from build123d import *

# Parameters (mm, degrees)
F0_R     = 1.4605
F1_DEPTH = 6.35


# Not quite as in the source:
# - a feature names something its author has since deleted; it is built from what else it names


with BuildPart() as f1:
    # F0 (on Top) → F1 (new body)
    with BuildSketch(Plane.XY):
        Polygon((76.2, 19.05), (76.2, 35.8597988734), (-76.2, 35.8597988734), (-76.2, 21.2902011266), (-73.2282, 21.2902011266), (-73.2282, 1.4605), (-65.6082, 1.4605), (-65.6082, 3.175), (-63.1952, 3.175), (-63.1952, 1.4605), (-55.5752, 1.4605), (-55.5752, -1.4605), (-63.1952, -1.4605), (-63.1952, -3.175), (-65.6082, -3.175), (-65.6082, -1.4605), (-73.2282, -1.4605), (-73.2282, -16.8097988734), (-76.2, -16.8097988734), (-76.2, -35.8597988734), (-57.15, -35.8597988734), (-57.15, -38.8315988734), (-19.05, -38.8315988734), (-19.05, -35.8597988734), (-1.4605, -35.8597988734), (-1.4605, -28.2397988734), (-3.175, -28.2397988734), (-3.175, -25.8267988734), (-1.4605, -25.8267988734), (-1.4605, -18.2067988734), (1.4605, -18.2067988734), (1.4605, -25.8267988734), (3.175, -25.8267988734), (3.175, -28.2397988734), (1.4605, -28.2397988734), (1.4605, -35.8597988734), (19.05, -35.8597988734), (19.05, -38.8315988734), (57.15, -38.8315988734), (57.15, -36.9798994367), (57.15, -35.8597988734), (76.2, -35.8597988734), (76.2, -19.05), (73.2282, -19.05), (73.2282, -1.4605), (65.6082, -1.4605), (65.6082, -3.175), (63.1952, -3.175), (63.1952, -1.4605), (55.5752, -1.4605), (55.5752, 1.4605), (63.1952, 1.4605), (63.1952, 3.175), (65.6082, 3.175), (65.6082, 1.4605), (73.2282, 1.4605), (73.2282, 19.05), align=None)
        with Locations((-38.1, -37.3456988734)):
            Circle(F0_R, mode=Mode.SUBTRACT)
        with BuildLine():
            ThreePointArc((39.5605, -37.3456988734), (39.5181253393, -37.6949563314), (39.3934602575, -38.0239472145))
            ThreePointArc((39.3934602575, -38.0239472145), (36.6818746607, -36.9964414154), (39.5605, -37.3456988734))
        make_face(mode=Mode.SUBTRACT)
        with BuildLine():
            add(Edge.make_bspline(
                [(-21.3872035351, 27.8586064071), (-20.0222567073, 26.4936595793), (-20.0222567073, 24.0434586691)],
                knots=[0, 0, 0, 1, 1, 1], degree=2))
            add(Edge.make_bspline(
                [(-20.0222567073, 24.0434586691), (-20.0222567073, 21.4291405282), (-21.441524027, 20.0457016181)],
                knots=[0, 0, 0, 1, 1, 1], degree=2))
            add(Edge.make_bspline(
                [(-21.441524027, 20.0457016181), (-22.8607913466, 18.6622627079), (-25.525962714, 18.6622627079)],
                knots=[0, 0, 0, 1, 1, 1], degree=2))
            Line((-25.525962714, 18.6622627079), (-28.4523347444, 18.6622627079))
            Line((-28.4523347444, 18.6622627079), (-28.4523347444, 29.2235532349))
            Line((-28.4523347444, 29.2235532349), (-25.2162203348, 29.2235532349))
            add(Edge.make_bspline(
                [(-25.2162203348, 29.2235532349), (-22.7521503629, 29.2235532349), (-21.3872035351, 27.8586064071)],
                knots=[0, 0, 0, 1, 1, 1], degree=2))
        make_face(mode=Mode.SUBTRACT)
        Polygon((-11.2662557189, 19.7740991587), (-11.2662557189, 18.6622627079), (-18.526709548, 18.6622627079), (-18.526709548, 19.6238509897), (-12.9212970884, 28.118651315), (-18.353346276, 28.118651315), (-18.353346276, 29.2235532349), (-11.4257499291, 29.2235532349), (-11.4257499291, 28.2619649531), (-17.0311623887, 19.7740991587), align=None, mode=Mode.SUBTRACT)
        Polygon((57.15, -36.9798994367), (76.2, -35.8597988734), (57.15, -35.8597988734), align=None)
    extrude(amount=F1_DEPTH)


solid = f1.part
CAD build for the part. Positions are in the model's coordinates, mm. A direction names the side the tool comes from. Round coordinates to 2 decimals unless told otherwise and drop trailing zeros. Write each loop counter-clockwise with the first axis right and the second up, starting at its lowest first coordinate (ties: lowest second). Pieces come first, ordered by that corner, then holes.
(1) Drop flat-ended pins along their axis: P1, Ø1.5, axis at x = 10.5, z = 3, coming from the -Y side; P2, Ø0.9, axis at x = 0.5, z = 4, coming from the -Y side; P3, Ø1.9, axis at y = -2.5, z = 3, coming from the +X side. Give the stop position or say it passes through.
(2) Slice it at D-D, the plane x = -6. Write the cut outline in (y, z).
(3) Probe line 1 along X through (y, z) = (-31, 2.25); line 2 along X through (y, z) = (28, 5); line 3 along Y through (x, z) = (-27, 1.5). List the from-to ranges inside material, lowest first.
(4) Slice it at B-B, the plane z = 4.25. Count the separate pieces of the cut face and the enclosed holes in it, and give its area (3 significant figures).
(5) 3-axis set-ups, long thin cutter, end or side, ignore diameter. For faces 5 (the face through (-14, 19.774, 3)), 6 (the face through (-57.15, -37, 3)), 7 (the face through (75, 19.05, 3)), 8 (the face through (-69, 1.46, 3)), 9 (the face through (1.46, -32, 3)): which of +Z, -Z, +X, -X, +Y, -Y reach the whole face in a straight line?
(6) Mould opens along Y. For faces 1 (the face through (-75, 21.29, 3)), 2 (the face through (10, -35.86, 3)), 3 (the face through (-76.2, -26, 3)), 4 (the face through (-15, 18.662, 3)) say: pulls with the +Y half, pulls with the -Y half, needs draft (parallel to the pull), parting line crosses it, or undercut.
(7) Slice it at C-C, the plane y = 6. Write the cut outline in (x, z), and give its area (3 significant figures).
From the geometry:
1. P1: stops at y = -35.86
1. P2: stops at y = -18.21
1. P3: stops at x = 73.23
2. outline: (-35.86, 0) - (35.86, 0) - (35.86, 6.35) - (-35.86, 6.35) - close
3. line 1: x = -76.2 to -1.46, 1.46 to 76.2
3. line 2: x = -76.2 to -28.45, -21.54 to -13, -11.6 to 76.2
3. line 3: y = -38.83 to 18.66, 29.22 to 35.86
4. separate pieces: 1
4. enclosed holes: 4
4. area: 10,600 mm2
5. face 5: +Z, -Z
5. face 6: +Z, -Z, -X, -Y
5. face 7: +Z, -Z, +X
5. face 8: +Z, -Z, -X
5. face 9: +Z, -Z, -Y
6. face 1: undercut
6. face 2: pulls with the -Y half
6. face 3: needs draft
6. face 4: undercut
7. outline: (-73.23, 0) - (73.23, 0) - (73.23, 6.35) - (-73.23, 6.35) - close
7. area: 930 mm2
